Design review of the part built by this model. Coordinates are the model's own, in mm. Give positions to 0.01 mm unless a question says otherwise; leave off trailing zeros. Order: outer loops, then holes, each group sorted by start corner. A loop starts at its lowest first (then second) coordinate and runs counter-clockwise, first axis right, second up. Notation, with made-up numbers: (61, 11.25) -> (66, 11.25) arc R27 ccw to (66, 50.25) -> close; hole circle Ø2 at (3.5, -23). An arc over 180 degrees is marked (long way). One line per item, written item: value.
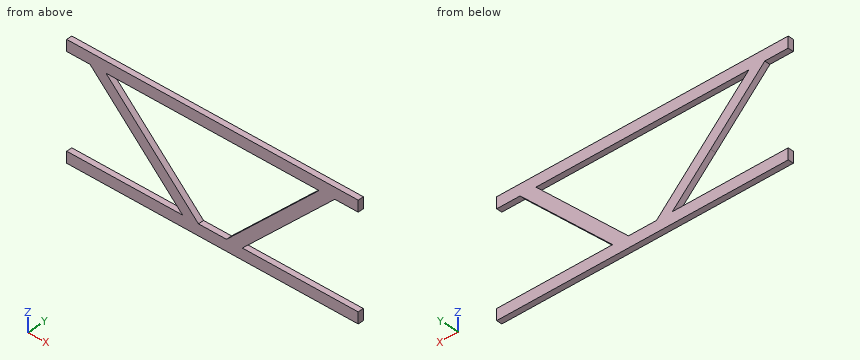
from build123d import *

# Parameters (mm, degrees)
F1_DEPTH = 25.4


with BuildPart() as f1:
    # F0 (on Front) → F1 (new body)
    with BuildSketch(Plane.XZ):
        Polygon((660.4, 209.55), (660.4, 260.35), (-660.4, 260.35), (-660.4, 209.55), (-554.442049, 209.55), (-482.6, 209.55), (-63.5, 209.55), (63.5, 209.55), (482.6, 209.55), (554.442049, 209.55), align=None)
        Polygon((308.971024, -35.921024), (554.442049, 209.55), (482.6, 209.55), (63.5, -209.55), (135.342049, -209.55), align=None)
        Polygon((135.342049, -209.55), (63.5, -209.55), (-63.5, -209.55), (-135.342049, -209.55), (-660.4, -209.55), (-660.4, -260.35), (660.4, -260.35), (660.4, -209.55), align=None)
        Polygon((-482.6, 209.55), (-554.442049, 209.55), (-308.971024, -35.921024), (-135.342049, -209.55), (-63.5, -209.55), align=None)
    extrude(amount=F1_DEPTH)


solid = f1.part
Item 1: Add section A-A on x = 121.5. Give the boundary of the cut face in (y, z), plus the area to 3 significant figures.
Returned:
outline: (-25.4, -260.35) -> (0, -260.35) -> (0, -151.55) -> (-25.4, -151.55) -> close; (-25.4, 209.55) -> (0, 209.55) -> (0, 260.35) -> (-25.4, 260.35) -> close
area: 4,050 mm²
Item 2: Clearance check with flat-ended pins moving along their axes: P1, Ø2, axis at y = -14.5, z = -29, coming from the -X side; P2, Ø1, axis at y = -15, z = -42, coming from the -X side; P3, Ø5, axis at y = -4.5, z = 25, coming from the -X side. State where each tip first meets the part, or that it passes through.
Returned:
P1: x = -316.89
P2: x = -303.39
P3: x = -372.39
Item 3: Add section D-D on x = 270.5. Give the boundary of the cut face in (y, z), plus the area to 3 significant figures.
Returned:
outline: (-25.4, -260.35) -> (0, -260.35) -> (0, -209.55) -> (-25.4, -209.55) -> close; (-25.4, -74.39) -> (0, -74.39) -> (0, -2.55) -> (-25.4, -2.55) -> close; (-25.4, 209.55) -> (0, 209.55) -> (0, 260.35) -> (-25.4, 260.35) -> close
area: 4,410 mm²
Item 4: Add section B-B on y = -20.25. Give the boundary of the cut face in (x, z).
Returned:
outline: (-660.4, -260.35) -> (660.4, -260.35) -> (660.4, -209.55) -> (135.34, -209.55) -> (554.44, 209.55) -> (660.4, 209.55) -> (660.4, 260.35) -> (-660.4, 260.35) -> (-660.4, 209.55) -> (-554.44, 209.55) -> (-135.34, -209.55) -> (-660.4, -209.55) -> close; hole (-482.6, 209.55) -> (-63.5, -209.55) -> (63.5, -209.55) -> (482.6, 209.55) -> close
Item 5: To check wall thickness, follow line 1 along Z through (x, y) = (-58, -1.25); line 2 along Z through (x, y) = (-185, -15.75); line 3 along Z through (x, y) = (279, -5.25). State the ranges of each line that lie inside material, in increasing order. Write a range as from..to.
Returned:
line 1: -260.35..-209.55, 209.55..260.35
line 2: -260.35..-209.55, -159.89..-88.05, 209.55..260.35
line 3: -260.35..-209.55, -65.89..5.95, 209.55..260.35
Item 6: Add section C-C on z = 32.5. Give the boundary of the cut face in (x, y), plus the area to 3 significant figures.
Returned:
outline: (-377.39, -25.4) -> (-305.55, -25.4) -> (-305.55, 0) -> (-377.39, 0) -> close; (305.55, -25.4) -> (377.39, -25.4) -> (377.39, 0) -> (305.55, 0) -> close
area: 3,650 mm²
